For this review, take the finished solid that the model builds, in its own axes (mm). Face numbers are marked on the shaded views. A direction names the side the tool comes from. Round coordinates to 2 decimals unless told otherwise and drop trailing zeros. Write each loop counter-clockwise with the first axis right and the second up, starting at its lowest first coordinate (ties: lowest second). Pieces come first, ordered by that corner, then holes.
Autodesk Inventor part; units mm, degrees
ref_plane "YZ Plane" through (0, 0, 0) normal (1, 0, 0) x (0, 1, 0)
ref_plane "XZ Plane" through (0, 0, 0) normal (0, 1, 0) x (-1, 0, 0)
ref_plane "XY Plane" through (0, 0, 0) normal (0, 0, 1) x (1, 0, 0)
sketch "Sketch1" plane through (0, 0, 0) normal (0, 0, 1) x (1, 0, 0)
  line L0 (0, -1.0008) -> (0, 6.0046) construction
  line L1 (-0.4047, 5.0038) -> (-1.5018, 1.9384)
  line L2 (-1.6213, 1.8542) -> (-1.9177, 1.8542)
  line L3 (-2.0447, 1.7272) -> (-2.0447, 0.9652)
  line L4 (-2.1717, 0.8382) -> (-2.794, 0.8382)
  line L5 (-2.794, 0.8382) -> (-2.794, 0)
  line L6 (-2.794, 0) -> (-1.397, 0)
  line L7 (-1.397, 0) -> (-1.397, 1.6002)
  arc A0 (-1.397, 1.6002) -> (-1.1579, 1.7686) centre (-1.397, 1.8542) ccw
  line L8 (-1.1579, 1.7686) -> (0, 5.0038)
  line L9 (-0.4047, 5.0038) -> (0, 5.0038)
  arc A1 (-1.6213, 1.8542) -> (-1.5018, 1.9384) centre (-1.6213, 1.9812) ccw
  arc A2 (-1.9177, 1.8542) -> (-2.0447, 1.7272) centre (-1.9177, 1.7272) ccw
  arc A3 (-2.1717, 0.8382) -> (-2.0447, 0.9652) centre (-2.1717, 0.9652) ccw
  line L10 (-1.7907, 5.0038) -> (-1.7907, 1.9812)
  arc A4 (-1.9177, 1.8542) -> (-1.7907, 1.9812) centre (-1.9177, 1.9812) ccw
  line L11 (-1.7907, 5.0038) -> (-0.4047, 5.0038)
  point P0 (0, 0)
  dimension "d0" = 5.588
  dimension "d1" = 0.8382
  dimension "d2" = 4.0894
  dimension "d5" = 0.381
  dimension "d7" = 0.127
  dimension "d8" = 5.0038
  dimension "d9" = 1.016
  dimension "d10" = 0.254
  dimension "d11" = 0.254
  dimension "d18" = 2.794
revolve "Revolution1" add sketch "Sketch1" angle 360 about axis through (0, -10, 0) along (0, 1, 0)
extrude "Extrusion1" cut sketch "Sketch1" along normal through all both and the other way through all contours L1 A1 L2 A4 L10 L11
mirror "Mirror1" about plane through (0, 0, 0) normal (1, 0, 0) of "Extrusion1"
sketch "Sketch2" plane through (-0.4047, 5.0038, 1.7444) normal (0, 1, 0) x (1, 0, 0)
  line L0 (0.4047, 3.2277) -> (0.4047, 0.261) construction
  line L1 (0.4034, 3.2277) -> (0.4059, 3.2277)
  line L2 (0.4059, 3.2277) -> (0.4059, 0.261)
  line L3 (0.4059, 0.261) -> (0.4034, 0.261)
  line L4 (0.4034, 0.261) -> (0.4034, 3.2277)
  point P0 (0.4047, 1.7444)
  dimension "d15" = 0.0025
extrude "Extrusion2" cut sketch "Sketch2" against normal blind 0.0254
properties part number "DU039.005-952.01" material "ML952 REZLYN"
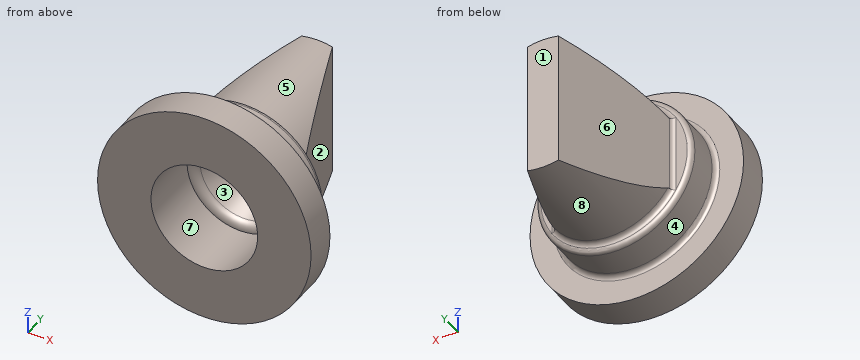
(1) For pin 1 Ø1.5 at (y, z) = (1, -1.5) entering from +X; pin 2 Ø3 at (x, y) = (0, 2.5) entering from -Z, all flat-tipped, find the tip position at first contact; note any pin that passes through.
Geometry check:
pin 1: stops at x = 2.69
pin 2: stops at z = -2.04
(2) We need section D-D, the plane y = 3.1. Give the boundary of the cut face in (x, z).
Geometry check:
outline: (-1.09, -1.42) arc R1.79 ccw to (1.09, -1.42) - (1.09, 1.42) arc R1.79 ccw to (-1.09, 1.42) - close; hole circle Ø1.36 at (0, 0)
(3) We need section B-B, the plane y = 0.6. Give the boundary of the cut face in (x, z).
Geometry check:
outline: circle Ø5.59 at (0, 0); hole circle Ø2.79 at (0, 0)
(4) For line 1 along Z through (x, y) = (0, 0.3); line 2 along Z through (x, y) = (0, 1.2); line 3 along Y through (x, z) = (2.2, -1.2), list the stretches that pass through material, from the lowest coordinate up.
Geometry check:
line 1: z = -2.79 to -1.4, 1.4 to 2.79
line 2: z = -2.04 to -1.4, 1.4 to 2.04
line 3: y = 0 to 0.84
(5) We need section A-A, the plane y = 1.15. Give the boundary of the cut face in (x, z).
Geometry check:
outline: circle Ø4.09 at (0, 0); hole circle Ø2.79 at (0, 0)
(6) We need section C-C, the plane y = 4.1. Give the boundary of the cut face in (x, z), and give its area (3 significant figures).
Geometry check:
outline: (-0.73, -1.64) arc R1.79 ccw to (0.73, -1.64) - (0.73, 1.64) arc R1.79 ccw to (-0.73, 1.64) - close; hole circle Ø0.65 at (0, 0)
area: 4.74 mm2
(7) Mouldability with a two-part tool opening along X and no side actions: class the marked faces 1, 2 and 3 as pulls with the +X half, pulls with the -X half, needs draft (parallel to the pull), parting line crosses it, or undercut.
Geometry check:
face 1: needs draft
face 2: pulls with the +X half
face 3: undercut
(8) For the marked faces 4, 5, 6, 7 and 8, list the 3-axis set-ups (+Z, -Z, +X, -X, +Y, -Y) from which the entire face can be reached by the end or side of a thin tool; tool diameter is ignored.
Geometry check:
face 4: +Y
face 5: +Z, +Y
face 6: +Z, -Z, -X, +Y
face 7: -Y
face 8: -Z, +Y
